```python
from build123d import *

# Parameters (mm, degrees)
BASE_FLANGIA1_DEPTH             = 1.5
BORDO_FLANGIA1_START            = -24
BORDO_FLANGIA1_OUTLINE_W        = 1.5
BORDO_FLANGIA1_OUTLINE_H        = 38.5
BORDO_FLANGIA1_DEPTH            = 15
BORDO_FLANGIA1_START_2          = -15
BORDO_FLANGIA1_2_OUTLINE_W      = 1.5
BORDO_FLANGIA1_2_OUTLINE_H      = 38.5
BORDO_FLANGIA1_2_DEPTH          = 15
BORDO_FLANGIA1_3_DEPTH          = 15
BORDO_FLANGIA1_4_DEPTH          = 15
FORO_FILETTATO_M8_1_D           = 6.8
FORO_FILETTATO_M8_1_ON_FACE_2_D = 6.8


# Read off the part's stored shape, not the designer's step: Schizzo10
# Sheet-metal steps are written as plain solids
with BuildPart() as part:
    # Schizzo1 → Base-Flangia1 (new body)
    with BuildSketch(Plane.XY):
        Polygon((0, 0), (0, 9), (-15, 9), (-15, -15), (24, -15), (24, 0), align=None)
    extrude(amount=-BASE_FLANGIA1_DEPTH)

    # Bordo-Flangia1 outline → Bordo-Flangia1 (add)
    with BuildSketch(Plane(origin=(0, 9, 0), x_dir=(-1, 0, 0), z_dir=(0, 1, 0)).offset(BORDO_FLANGIA1_START)):
        with Locations((-23.25, 19.25)):
            Rectangle(BORDO_FLANGIA1_OUTLINE_W, BORDO_FLANGIA1_OUTLINE_H)
    extrude(amount=BORDO_FLANGIA1_DEPTH)

    # Bordo-Flangia1 2 outline → Bordo-Flangia1 2 (add)
    with BuildSketch(Plane.YZ.offset(BORDO_FLANGIA1_START_2)):
        with Locations((8.25, 19.25)):
            Rectangle(BORDO_FLANGIA1_2_OUTLINE_W, BORDO_FLANGIA1_2_OUTLINE_H)
    extrude(amount=BORDO_FLANGIA1_2_DEPTH)

    # Bordo-Flangia1 3 outline → Bordo-Flangia1 3 (cut)
    with BuildSketch(Plane(origin=(0, 9, 0), x_dir=(-1, 0, 0), z_dir=(0, 1, 0)).offset(BORDO_FLANGIA1_START)):
        with BuildLine():
            ThreePointArc((-22.5, -1.5), (-23.560660172, -1.060660172), (-24, 0))
            Line((-24, 0), (-24, -1.5))
            Line((-24, -1.5), (-22.5, -1.5))
        make_face()
    extrude(amount=BORDO_FLANGIA1_3_DEPTH, mode=Mode.SUBTRACT)

    # Bordo-Flangia1 4 outline → Bordo-Flangia1 4 (cut)
    with BuildSketch(Plane.YZ.offset(BORDO_FLANGIA1_START_2)):
        with BuildLine():
            ThreePointArc((9, 0), (8.560660172, -1.060660172), (7.5, -1.5))
            Line((7.5, -1.5), (9, -1.5))
            Line((9, -1.5), (9, 0))
        make_face()
    extrude(amount=BORDO_FLANGIA1_4_DEPTH, mode=Mode.SUBTRACT)

    # Foro filettato M8-1 (through all)
    with Locations(Plane(origin=(-7.5, 9, 28.5), x_dir=(0, 0, 1), z_dir=(0, 1, 0))):
        with Locations((0, 0)):
            Hole(FORO_FILETTATO_M8_1_D / 2)

    # Foro filettato M8-1 on face 2 (through all)
    with Locations(Plane(origin=(24, -7.5, 28.5), x_dir=(0, 0, 1), z_dir=(1, 0, 0))):
        with Locations((0, 0)):
            Hole(FORO_FILETTATO_M8_1_ON_FACE_2_D / 2)


solid = part.part
```
Check sheet for the modelled part. Datum: model origin and axes. Units: mm. A direction names the side the tool comes from. Give positions to 0.01 mm unless a question says otherwise; leave off trailing zeros. Loops run counter-clockwise (first coordinate to the right, second up) from the corner with the lowest first, then second, coordinate; pieces in that order, holes last. Notation, with made-up numbers: (60.5, 32) - (69.5, 32) arc R25 ccw to (69.5, 58) - close; hole circle Ø10 at (70, 43). An arc over 180 degrees is marked (long way). One line per question, with ' | ' between items. Start each with the question number.
1. Cross-section at A-A, the plane y = -7.5. Enter the section's corners in (x, z).
2. Cross-section at B-B, the plane x = -7.5. Enter the section's corners in (y, z), plus the area to 3 significant figures.
3. Cross-section at D-D, the plane z = 1. Enter the section's corners in (x, y), plus the area to 3 significant figures.
4. Draft check along Z on faces 1 (the flat face through (22.5, -8, 19)), 2 (the cylindrical face through (-7.6, 8.57, -1.05)), 3 (the cylindrical face through (23.24, -8.521, 25.257)). Enter one of: released by +Z, released by -Z, zero draft, split by the parting line, or undercut.
5. Gauge pin test, flat ends, axial feed: pin 1 Ø6 at (x, y) = (-9.5, -7.5) entering from +Z; pin 2 Ø9 at (y, z) = (-7.5, 28.5) entering from -X; pin 3 Ø4.5 at (x, z) = (-10.5, 10) entering from -Y; pin 4 Ø6 at (x, z) = (-7.5, 28.5) entering from -Y. Record the tip position at first contact, or that the pin passes through.
6. Set-up check for faces 4 (the flat face through (3, -6, 0)), 5 (the flat face through (-8, 9, 19)), 6 (the flat face through (23, 0, 13)), 7 (the flat face through (23, -8, 38.5)), 8 (the flat face through (-8, 7.5, 19)): record each of +Z, -Z, +X, -X, +Y, -Y from which the full face is reachable in a straight line by a thin tool's end or side.
7. Cross-section at C-C, the plane z = 28.5. Enter the section's corners in (x, y).
8. Material ranges on line 1 along Y through (x, z) = (23.1, 28.5); line 2 along Z through (x, y) = (-1.5, -9); line 3 along X through (y, z) = (-4, 8.5), recorded low to high. Write a range as [from, to].
Check result:
1) outline: (-15, -1.5) - (22.5, -1.5) arc R1.5 ccw to (24, 0) - (24, 25.1) - (22.5, 25.1) - (22.5, 0) - (-15, 0) - close; (22.5, 31.9) - (24, 31.9) - (24, 38.5) - (22.5, 38.5) - close
2) outline: (-15, -1.5) - (7.5, -1.5) arc R1.5 ccw to (9, 0) - (9, 25.1) - (7.5, 25.1) - (7.5, 0) - (-15, 0) - close; (7.5, 31.9) - (9, 31.9) - (9, 38.5) - (7.5, 38.5) - close | area: 83.1 mm2
3) outline: (-15, 7.5) - (0, 7.5) - (0, 9) - (-15, 9) - close; (22.5, -15) - (24, -15) - (24, 0) - (22.5, 0) - close | area: 45.0 mm2
4) face 1: zero draft | face 2: released by -Z | face 3: undercut
5) pin 1: stops at z = 0 | pin 2: stops at x = 22.5 | pin 3: stops at y = 7.5 | pin 4: passes through
6) face 4: +Z, -X, -Y | face 5: +Z, -Z, +X, -X, +Y | face 6: +Z, -Z, +X, +Y | face 7: +Z, +X, -X, +Y, -Y | face 8: +Z, +X, -X, -Y
7) outline: (-15, 7.5) - (-10.9, 7.5) - (-10.9, 9) - (-15, 9) - close; (-4.1, 7.5) - (0, 7.5) - (0, 9) - (-4.1, 9) - close; (22.5, -15) - (24, -15) - (24, -10.9) - (22.5, -10.9) - close; (22.5, -4.1) - (24, -4.1) - (24, 0) - (22.5, 0) - close
8) line 1: y = [-15, -10.9], [-4.1, 0] | line 2: z = [-1.5, 0] | line 3: x = [22.5, 24]
